Geometry check sheet. Reference: drawing and pictorial views, mm from the part's lowest x, y, z. Coordinates: 2 decimals unless noted, no trailing zeros. Loops run counter-clockwise (first coordinate to the right, second up) from the corner with the lowest first, then second, coordinate; pieces in that order, holes last. Notation, with made-up numbers: (56.5, 24) -> (61.5, 24) arc R26 cw to (61.5, 38) -> close; hole circle Ø2 at (-28.5, -17). An arc over 180 degrees is marked (long way). Answer as a JSON object with one key per item and string values. Group by question number.
Q1. Scan lines: L1, parallel to X at y = 0.65, z = 16; L2, parallel to X at y = 9.25, z = 16; L3, parallel to Y at x = 3, z = 20.5. Record each from-to range of solid material in increasing order.
Q2. Cross-section at A-A on x = 16. Record the boundary of the cut face in (y, z).
Q3. Cross-section at D-D on x = 27.5. Record the boundary of the cut face in (y, z), and give its area (3 significant figures).
Q4. Cross-section at B-B on z = 16. Record the boundary of the cut face in (x, y), and give its area (3 significant figures).
Q5. Release check for a two-part mould opening along X. For the marked faces 1, 2 and 3 record: released by +X, released by -X, zero draft, split by the parting line, or undercut.
Q6. Gauge pin test, flat ends, axial feed: pin 1 Ø5 at (x, z) = (16, 27.5) entering from +Y; pin 2 Ø9 at (x, z) = (17, 15.5) entering from +Y; pin 3 Ø6 at (y, z) = (2.5, 25.5) entering from +X; pin 4 Ø4 at (x, y) = (28.5, 2.5) entering from +Z. Record the tip position at first contact, or that the pin passes through.
Q7. Cross-section at C-C on y = 6.75. Record the boundary of the cut face in (x, z), and give its area (3 significant figures).
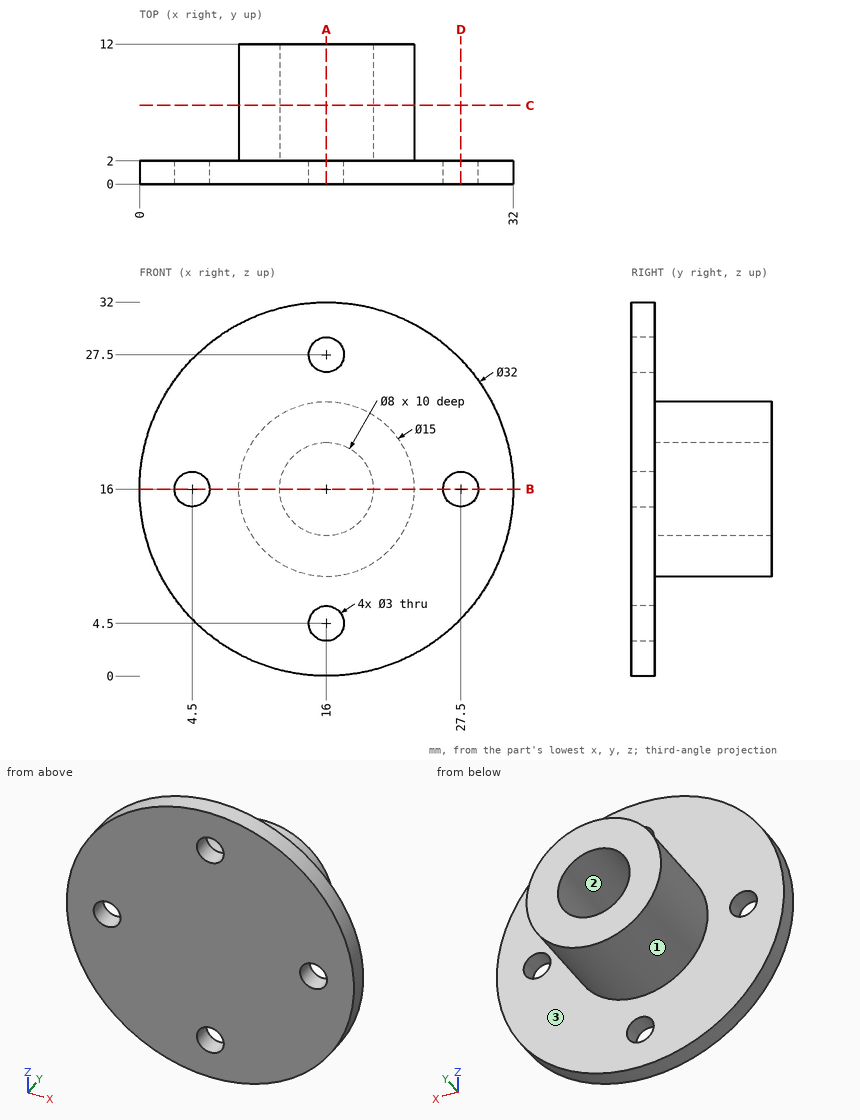
Computed values:
{
 "1": {"L1": "x = 0 to 3, 6 to 26, 29 to 32", "L2": "x = 8.5 to 12, 20 to 23.5", "L3": "y = 0 to 2"},
 "2": {"outline": "(0, 0) -> (2, 0) -> (2, 3) -> (0, 3) -> close; (0, 6) -> (2, 6) -> (2, 8.5) -> (12, 8.5) -> (12, 12) -> (2, 12) -> (2, 20) -> (12, 20) -> (12, 23.5) -> (2, 23.5) -> (2, 26) -> (0, 26) -> close; (0, 29) -> (2, 29) -> (2, 32) -> (0, 32) -> close"},
 "3": {"outline": "(0, 4.88) -> (2, 4.88) -> (2, 14.5) -> (0, 14.5) -> close; (0, 17.5) -> (2, 17.5) -> (2, 27.12) -> (0, 27.12) -> close", "area": "38.5 mm²"},
 "4": {"outline": "(0, 0) -> (3, 0) -> (3, 2) -> (0, 2) -> close; (6, 0) -> (26, 0) -> (26, 2) -> (23.5, 2) -> (23.5, 12) -> (20, 12) -> (20, 2) -> (12, 2) -> (12, 12) -> (8.5, 12) -> (8.5, 2) -> (6, 2) -> close; (29, 0) -> (32, 0) -> (32, 2) -> (29, 2) -> close", "area": "122 mm²"},
 "5": {"face 1": "split by the parting line", "face 2": "undercut", "face 3": "zero draft"},
 "6": {"pin 1": "stops at y = 2", "pin 2": "stops at y = 12", "pin 3": "stops at x = 30.6", "pin 4": "stops at z = 28.02"},
 "7": {"outline": "circle Ø15 at (16, 16); hole circle Ø8 at (16, 16)", "area": "126 mm²"}
}
